Verification items for the finished model (mm, model axes). Coordinates: 2 decimals unless noted, no trailing zeros. Order: outer loops, then holes, each group sorted by start corner. A loop starts at its lowest first (then second) coordinate and runs counter-clockwise, first axis right, second up. Notation, with made-up numbers: M 79.25,35 L 98.25,35 A7 cw 98.25,46 Z; hole C 17.5,-39 d8. An arc over 180 degrees is marked long. Return JSON: item names as keys, results as strings. Group by question number.
Q1. Section check C-C, the plane x = -5.75. Enter the section's corners in (y, z) (3 decimals), then the cut area to 3 significant figures.
Q2. Section check D-D, the plane z = -10. Enter the section's corners in (x, y) (3 decimals).
Q3. Go/stop test with flat-tipped pins: pin 1 Ø4.5 at (x, z) = (-10.5, 21) entering from +Y (3 decimals); pin 2 Ø2 at (x, z) = (-10.5, -22.5) entering from +Y. Record where each tip stops, or that it passes through.
Q4. Thickness scan on probe 1 along X at (y, z) = (2.05, -10); probe 2 along X at (y, z) = (0.85, -22.5); probe 3 along Z at (x, y) = (-5.5, 0.95). Record the ranges inside material, lowest first.
Q5. Section check A-A, the plane z = 21. Enter the section's corners in (x, y) (3 decimals), then the cut area to 3 significant figures.
Q6. Section check B-B, the plane y = 1.35. Count the separate pieces of the cut face and the enclosed holes in it, then the cut area to 3 significant figures.
from build123d import *

# Parameters (mm, degrees)
SKETCH1_W           = 30
SKETCH1_H           = 50
SKETCH1_R           = 1.25
SKETCH1_R_2         = 1.65
SKETCH1_W_2         = 8.169972816
SKETCH1_H_2         = 0.75
SKETCH1_W_3         = 9
SKETCH1_H_3         = 9
BOSS_EXTRUDE1_DEPTH = 3.175


with BuildPart() as part:
    # Sketch1 → Boss-Extrude1 (new body)
    with BuildSketch(Plane(origin=(0, 0, 0), x_dir=(1, 0, 0), z_dir=(0, 1, 0))):
        Rectangle(SKETCH1_W, SKETCH1_H)
        with Locations((-10.5, 22.5)):
            Circle(SKETCH1_R, mode=Mode.SUBTRACT)
        with Locations((10.5, 22.5)):
            Circle(SKETCH1_R, mode=Mode.SUBTRACT)
        with Locations((10.5, 10)):
            Circle(SKETCH1_R, mode=Mode.SUBTRACT)
        with Locations((-10.5, 10)):
            Circle(SKETCH1_R, mode=Mode.SUBTRACT)
        with Locations((-10.5, -21)):
            Circle(SKETCH1_R_2, mode=Mode.SUBTRACT)
        with Locations((10.5, -21)):
            Circle(SKETCH1_R_2, mode=Mode.SUBTRACT)
        with Locations((6.415013592, -10.275512249)):
            Rectangle(SKETCH1_W_2, SKETCH1_H_2, mode=Mode.SUBTRACT)
        with Locations((-6.415013592, -12.525512249)):
            Rectangle(SKETCH1_W_2, SKETCH1_H_2, mode=Mode.SUBTRACT)
        with Locations((-6.415013592, -10.275512249)):
            Rectangle(SKETCH1_W_2, SKETCH1_H_2, mode=Mode.SUBTRACT)
        with Locations((6.415013592, -12.525512249)):
            Rectangle(SKETCH1_W_2, SKETCH1_H_2, mode=Mode.SUBTRACT)
        with Locations((0, 10)):
            Rectangle(SKETCH1_W_3, SKETCH1_H_3, mode=Mode.SUBTRACT)
    extrude(amount=BOSS_EXTRUDE1_DEPTH)


solid = part.part
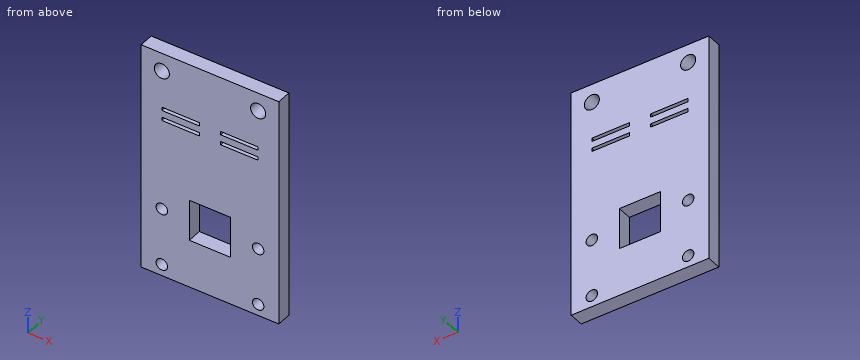
Numbers:
{
 "1": {"outline": "M 0,-25 L 3.175,-25 L 3.175,9.901 L 0,9.901 Z; M 0,10.651 L 3.175,10.651 L 3.175,12.151 L 0,12.151 Z; M 0,12.901 L 3.175,12.901 L 3.175,25 L 0,25 Z", "area": "154 mm2"},
 "2": {"outline": "M -15,0 L -11.75,0 L -11.75,3.175 L -15,3.175 Z; M -9.25,0 L -4.5,0 L -4.5,3.175 L -9.25,3.175 Z; M 4.5,0 L 9.25,0 L 9.25,3.175 L 4.5,3.175 Z; M 11.75,0 L 15,0 L 15,3.175 L 11.75,3.175 Z"},
 "3": {"pin 1": "stops at y = 3.175", "pin 2": "passes through"},
 "4": {"probe 1": "x = -15 to -11.75, -9.25 to -4.5, 4.5 to 9.25, 11.75 to 15", "probe 2": "x = -15 to -11.75, -9.25 to 9.25, 11.75 to 15", "probe 3": "z = -25 to 9.9, 10.65 to 12.15, 12.9 to 25"},
 "5": {"outline": "M -15,0 L -12.15,0 L -12.15,3.175 L -15,3.175 Z; M -8.85,0 L 8.85,0 L 8.85,3.175 L -8.85,3.175 Z; M 12.15,0 L 15,0 L 15,3.175 L 12.15,3.175 Z", "area": "74.3 mm2"},
 "6": {"separate pieces": "1", "enclosed holes": "11", "area": "1,360 mm2"}
}
